Job drawing, mm, ordinate dimensions from the low corner. One solid piece. A direction names the side the tool comes from. Give positions to 0.01 mm unless a question says otherwise; leave off trailing zeros. Order: outer loops, then holes, each group sorted by start corner. A loop starts at its lowest first (then second) coordinate and runs counter-clockwise, first axis right, second up. Notation, with made-up numbers: (77.5, -2.75) - (95.5, -2.75) arc R28 cw to (95.5, 25.25) - close; hole circle Ø7 at (-13, -5.5). An arc over 180 degrees is marked (long way). Write each question's results on one line, items separated by ' | '. Start each with the question number.
1) Cut at B-B on x = 22. List the corners of the cut face in (y, z), plus the area to 3 significant figures.
2) Cut at A-A on z = 39. List the corners of the cut face in (x, y).
3) Cut at D-D on z = 12. List the corners of the cut face in (x, y).
4) Tool access for the marked faces 1 and 2: list every direction of +Z, -Z, +X, -X, +Y, -Y with a clear straight run to the whole face (end or side of a thin tool).
5) Cut at C-C on y = 2.25. List the corners of the cut face in (x, z).
6) Drill centre lines: line 1 along Y through (x, z) = (34, 30.5); line 2 along X through (y, z) = (7.25, 5.5); line 3 along Z through (x, y) = (35.5, 11). Where is each one in solid material? Low to high. Write a range as from..to.
7) Drop a flat-ended pin along its axis: pin 1 Ø20 at (x, z) = (34, 25.5) entering from -Y. Give the stop position or say it passes through.
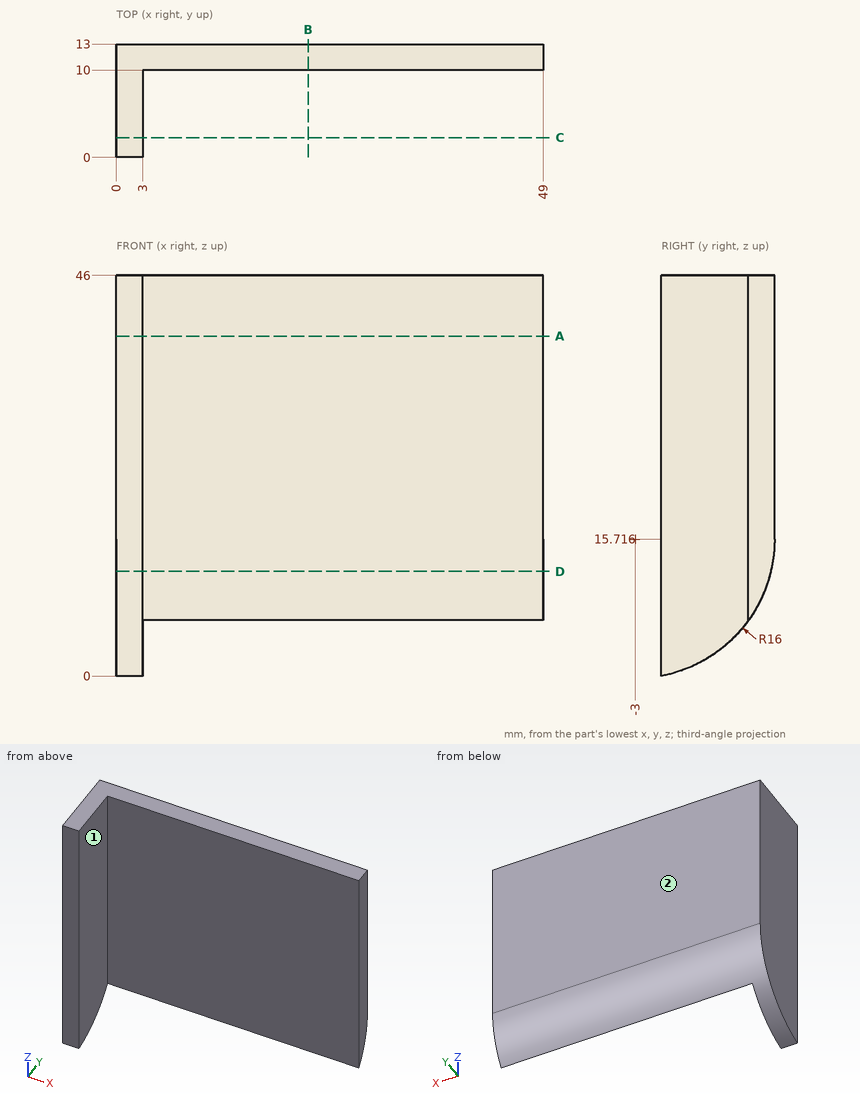
Results:
1) outline: (10, 6.39) arc R16 ccw to (13, 15.72) - (13, 46) - (10, 46) - close | area: 110 mm^2
2) outline: (0, 0) - (3, 0) - (3, 10) - (49, 10) - (49, 13) - (0, 13) - close
3) outline: (0, 0) - (3, 0) - (3, 10) - (49, 10) - (49, 12.56) - (0, 12.56) - close
4) face 1: +Z, -Z, +X, -Y | face 2: +Z, -Z, +X, -X, +Y
5) outline: (0, 0.6) - (3, 0.6) - (3, 46) - (0, 46) - close
6) line 1: 10..13 | line 2: 0..3 | line 3: 7.97..46
7) pin 1: y = 10
